Autodesk Inventor part; units mm, degrees
ref_plane "YZ Plane" through (0, 0, 0) normal (1, 0, 0) x (0, 1, 0)
ref_plane "XZ Plane" through (0, 0, 0) normal (0, 1, 0) x (-1, 0, 0)
ref_plane "XY Plane" through (0, 0, 0) normal (0, 0, 1) x (1, 0, 0)
sketch "Sketch1" plane through (0, 0, 0) normal (1, 0, 0) x (0, 1, 0)
  line L0 (7, 0) -> (29.5, 0)
  line L1 (0, 0) -> (7, 0)
  line L2 (7, 0) -> (29.5, 0)
  line L3 (29.5, 0) -> (29.5, 15.8)
  line L4 (7, 15.8) -> (7, 0)
  line L5 (29.5, 15.8) -> (34.4, 15.8) construction
  line L6 (2.1, 15.8) -> (2.1, 18.2)
  line L7 (34.4, 18.2) -> (34.4, 15.8)
  line L8 (7, 18.2) -> (7, 22.5)
  line L9 (7, 22.5) -> (29.5, 22.5)
  line L10 (29.5, 22.5) -> (29.5, 18.2)
  line L11 (2.1, 18.2) -> (7, 18.2)
  line L12 (29.5, 18.2) -> (34.4, 18.2)
  line L13 (34.4, 15.8) -> (29.5, 15.8)
  line L14 (7, 15.8) -> (2.1, 15.8)
  dimension "d2" = 22.5
  dimension "d3" = 15.8
  dimension "d5" = 2.4
  dimension "d6" = 4.3
  dimension "d7" = 22.5
  dimension "d8" = 4.3
  dimension "d9" = 2.4
  dimension "d10" = 15.8
  dimension "d13" = 4.9
  dimension "d14" = 4.9
extrude "Extrusion1" add sketch "Sketch1" along normal blind 12
sketch "Sketch2" plane through (0, 7, 22.5) normal (0, 0, 1) x (1, 0, 0)
  line L0 (0, 22.5) -> (0, 0)
  line L1 (0, 0) -> (12, 0)
  line L2 (12, 22.5) -> (12, 0)
  line L3 (0, 22.5) -> (12, 22.5)
  line L4 (0, 0) -> (12, 0)
  line L5 (0, -4.9) -> (12, -4.9)
  circle A0 centre (6, 6) radius 0.7 construction
  circle A1 centre (6, 6) radius 2.4 construction
  line L6 (0, 0) -> (12, 0)
  arc A2 (3.371, 11.3933) -> (8.629, 11.3933) centre (6, 6) ccw
  line L7 (12, 0) -> (12, 22.5)
  arc A3 (8.629, 11.3933) -> (3.371, 11.3933) centre (6, 12.2) ccw
  point P0 (0, -7)
  dimension "d16" = 1.4
  dimension "d17" = 4.8
  dimension "d20" = 5.5
  dimension "d21" = 6
  dimension "d22" = 6.2
extrude "Extrusion2" add sketch "Sketch2" along normal blind 4.3 contours A2 A3
sketch "Sketch3" plane through (0, 7, 26.8) normal (0, 0, 1) x (1, 0, 0)
  circle A0 centre (6, 6) radius 0.7
  circle A1 centre (6, 6) radius 2.4
  dimension "d25" = 1.4
  dimension "d26" = 4.8
extrude "Extrusion3" add sketch "Sketch3" along normal blind 2.9
sketch "Sketch4" plane through (0, 29.5, 18.2) normal (0, 0, 1) x (1, 0, 0)
  line L0 (0, -22.5) -> (0, -27.4)
  line L1 (0, -27.4) -> (12, -27.4)
  line L2 (12, -22.5) -> (12, -27.4)
  line L3 (0, -22.5) -> (12, -22.5)
  line L4 (0, 4.9) -> (0, 0)
  line L5 (0, 0) -> (12, 0)
  line L6 (12, 4.9) -> (12, 0)
  line L7 (0, 4.9) -> (12, 4.9)
  line L8 (0, -16.5) -> (0, -22.5)
  line L9 (0, 0) -> (0, -16.5)
  line L10 (12, 0) -> (12, -16.5)
  line L11 (12, -16.5) -> (12, -22.5)
  line L12 (0, -22.5) -> (0, 0)
  line L13 (0, -11.25) -> (12, -11.25)
  arc A0 (5.3, 4.9) -> (6.7, 4.9) centre (6, 4.3343) ccw
  line L14 (5.3, 4.9) -> (6.7, 4.9)
  line L15 (0, 4.9) -> (12, 4.9)
  arc A1 (6.7, -27.4) -> (5.3, -27.4) centre (6, -26.8343) ccw
  line L16 (5.3, -27.4) -> (6.7, -27.4)
  point P0 (0, -29.5)
  point P1 (5.3, -27.4)
  dimension "d32" = 5.3
  dimension "d33" = 5.3
  dimension "d35" = 0.9
extrude "Extrusion4" cut sketch "Sketch4" against normal up to surface (2.4 mm away) contours A1 L1 | L7 A0
properties part number "Microservo Mg90"
For this review, take the finished solid that the model builds, in its own axes (mm). A direction names the side the tool comes from. Round coordinates to 2 decimals unless told otherwise and drop trailing zeros. Write each loop counter-clockwise with the first axis right and the second up, starting at its lowest first coordinate (ties: lowest second). Pieces come first, ordered by that corner, then holes.
1) Machinability: for faces 5 (the face through (6, 29.5, 8)), 6 (the face through (6, 13, 26.8)), 7 (the face through (6, 7, 8)), which of the approach directions +Z, -Z, +X, -X, +Y, -Y give a long, thin tool a straight path to every point of the face, cutting with its end or side? Answer none if there is none.
Answer below:
face 5: -Z, +X, -X, +Y
face 6: +Z
face 7: -Z, +X, -X, -Y
2) Take a section at B-B on x = 9.75. Give the boundary of the cut face in (y, z).
Answer below:
outline: (2.1, 15.8) - (7, 15.8) - (7, 0) - (29.5, 0) - (29.5, 15.8) - (34.4, 15.8) - (34.4, 18.2) - (29.5, 18.2) - (29.5, 22.5) - (17.68, 22.5) - (17.68, 26.8) - (8.32, 26.8) - (8.32, 22.5) - (7, 22.5) - (7, 18.2) - (2.1, 18.2) - close
3) Mouldability with a two-part tool opening along X and no side actions: class faces 1 (the face through (5.972, 32.935, 17.017)), 2 (the face through (5.445, 13.426, 28.23)), 3 (the face through (5.69, 10.62, 28.23)), 4 (the face through (6, 29.5, 20)) as +X half, -X half, draft (parallel to the pull), parting line (faces both ways), or undercut.
Answer below:
face 1: undercut
face 2: undercut
face 3: parting line
face 4: draft
4) Take a section at D-D on y = 15. Give the boundary of the cut face in (x, z).
Answer below:
outline: (0, 0) - (12, 0) - (12, 22.5) - (11.66, 22.5) - (11.66, 26.8) - (7.33, 26.8) - (7.33, 29.7) - (4.67, 29.7) - (4.67, 26.8) - (0.34, 26.8) - (0.34, 22.5) - (0, 22.5) - close
5) Take a section at C-C on z = 4. Give the boundary of the cut face in (x, y), then the cut area to 3 significant figures.
Answer below:
outline: (0, 7) - (12, 7) - (12, 29.5) - (0, 29.5) - close
area: 270 mm2
6) For line 1 along Z through (x, y) = (1.25, 10); line 2 along Y through (x, z) = (6, 28.8); line 3 along Y through (x, z) = (6, 17.05), list the stretches that pass through material, from the lowest coordinate up.
Answer below:
line 1: z = 0 to 26.8
line 2: y = 10.6 to 12.3, 13.7 to 15.4
line 3: y = 3.57 to 32.93
7) Insertion check: pin 1 Ø2 at (x, z) = (9, 21.5) entering from +Y; pin 2 Ø5.5 at (x, y) = (5, 5) entering from +Z; pin 3 Ø1.3 at (x, z) = (7, 20.5) entering from -Y. Each pin has a flat end and moves straight along its axis. Give the tip position at first contact, or say it passes through.
Answer below:
pin 1: stops at y = 29.5
pin 2: stops at z = 26.8
pin 3: stops at y = 7
8) Take a section at A-A on y = 19.2. Give the boundary of the cut face in (x, z).
Answer below:
outline: (0, 0) - (12, 0) - (12, 22.5) - (8.75, 22.5) - (8.75, 26.8) - (3.25, 26.8) - (3.25, 22.5) - (0, 22.5) - close
